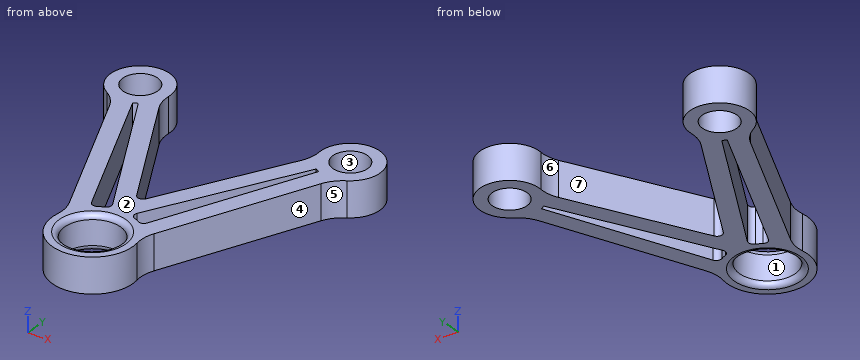
from build123d import *

# Parameters (mm, degrees)
SCHIZZO1_R                   = 5
SCHIZZO1_R_2                 = 8
ESTRUSIONE_ESTRUSIONE1_DEPTH = 5
RACCORDO1_R                  = 10
TAGLIO_ESTRUSIONE1_DEPTH     = 10
RACCORDO2_R                  = 1.5


with BuildPart() as part:
    # Schizzo1 → Estrusione-Estrusione1 (new body, symmetric)
    with BuildSketch(Plane.XY):
        with BuildLine():
            Line((-31.796659285, -8.307948929), (-10.655708964, -56.174972085))
            ThreePointArc((-10.655708964, -56.174972085), (0, -72), (10.655708964, -56.174972085))
            Line((10.655708964, -56.174972085), (31.796659285, -8.307948929))
            ThreePointArc((31.796659285, -8.307948929), (34.104135411, 7.443525544), (22.015418218, -2.914867709))
            Line((22.015418218, -2.914867709), (0, -43.668257767))
            Line((0, -43.668257767), (-22.015418218, -2.914867709))
            ThreePointArc((-22.015418218, -2.914867709), (-34.104135411, 7.443525544), (-31.796659285, -8.307948929))
        make_face()
        with Locations((-30, 0)):
            Circle(SCHIZZO1_R, mode=Mode.SUBTRACT)
        with Locations((30, 0)):
            Circle(SCHIZZO1_R, mode=Mode.SUBTRACT)
        with Locations((0, -60.5)):
            Circle(SCHIZZO1_R_2, mode=Mode.SUBTRACT)
    extrude(amount=ESTRUSIONE_ESTRUSIONE1_DEPTH, both=True)

    # Raccordo1
    raccordo1_edges = [part.edges().sort_by_distance(p)[0] for p in [
        (22.015418218, -2.914867709, 0),
        (31.796659285, -8.307948929, 0),
        (10.655708964, -56.174972085, 0),
        (-10.655708964, -56.174972085, 0),
        (-31.796659285, -8.307948929, 0),
        (-22.015418218, -2.914867709, 0),
    ]]
    fillet(raccordo1_edges, radius=RACCORDO1_R)

    # Schizzo2 → Taglio-Estrusione1 (cut)
    with BuildSketch(Plane.XY.offset(5)):
        with BuildLine():
            Line((-26.565911307, -7.775412198), (-7.229506839, -51.556609655))
            ThreePointArc((-7.229506839, -51.556609655), (-5.059978512, -50.173015084), (-2.637118885, -49.306448107))
            Line((-2.637118885, -49.306448107), (-25.408693659, -7.153314343))
            ThreePointArc((-25.408693659, -7.153314343), (-25.975264878, -7.486755452), (-26.565911307, -7.775412198))
        make_face()
        with BuildLine():
            Line((25.408693659, -7.153314343), (2.637118885, -49.306448107))
            ThreePointArc((2.637118885, -49.306448107), (5.059978512, -50.173015084), (7.229506839, -51.556609655))
            Line((7.229506839, -51.556609655), (26.565911307, -7.775412198))
            ThreePointArc((26.565911307, -7.775412198), (25.975264878, -7.486755452), (25.408693659, -7.153314343))
        make_face()
    extrude(amount=-TAGLIO_ESTRUSIONE1_DEPTH, mode=Mode.SUBTRACT)

    # Raccordo2
    raccordo2_edges = [part.edges().sort_by_distance(p)[0] for p in [
        (-8, -60.5, -5),
        (0, -43.668257767, 0),
        (-8, -60.5, 5),
        (7.229506839, -51.556609655, 0),
        (2.637118885, -49.306448107, 0),
        (-2.637118885, -49.306448107, 0),
        (-7.229506839, -51.556609655, 0),
    ]]
    fillet(raccordo2_edges, radius=RACCORDO2_R)


solid = part.part
Geometry: final body of the model. Coordinates: model frame, mm. Face numbers are marked on the shaded views. A direction names the side the tool comes from. Round coordinates to 2 decimals unless told otherwise and drop trailing zeros. Loops run counter-clockwise (first coordinate to the right, second up) from the corner with the lowest first, then second, coordinate; pieces in that order, holes last. Notation, with made-up numbers: (-37, -25.75) - (21, -25.75) arc R13 ccw to (21, -10.75) - close; hole circle Ø4 at (85.5, 31.5). An arc over 180 degrees is marked (long way). Write each question's results on one line, items separated by ' | '. Start each with the question number.
1) First-contact query: P1, Ø9.5, axis at x = 0, y = -60.5, coming from the -Z side; P2, Ø11.5, axis at x = -30, y = 0, coming from the -Z side; P3, Ø3, axis at y = -17.5, z = 3, coming from the +X side; P4, Ø5, axis at y = -15.5, z = -0.5, coming from the +X side. Flat tips, straight axial feed; report the tip coordinate or a pass-through.
2) Cut plane A-A on x = 0. Return loops of the section in (y, z).
3) Cut plane C-C on y = -40. Return loops of the section in (x, z).
4) Cut plane B-B on y = -60.5. Return loops of the section in (x, z), then the cut area to 3 significant figures.
5) Cut plane D-D on z = -0.25. Count the separate pieces of the cut face and the enclosed holes in it, then the cut area to 3 significant figures.
6) Mould query, pull axis Y, two halves, no side actions, for the marked faces 1, 2, 3 and 4. Classes: released by +Y, released by -Y, zero draft, split by the parting line, or undercut.
7) Access query for the marked faces 5, 6 and 7. Directions: +Z, -Z, +X, -X, +Y, -Y. A direction counts if a zero-diameter tool reaches every point of the face in a straight line with its end or side. Return the directions, or none.
8) Line query: probe 1 along X at (y, z) = (-14, 0); probe 2 along Y at (x, z) = (5, 0.5) (3 decimals); probe 3 along X at (y, z) = (-37, 2). Output: solid intervals per line, ascending. Write a range as [from, to].
Verdict:
1) P1: passes through | P2: stops at z = -5 | P3: stops at x = 28.4 | P4: stops at x = 29.72
2) outline: (-72, -5) - (-70, -5) arc R1.5 ccw to (-68.5, -3.5) - (-68.5, 3.5) arc R1.5 ccw to (-70, 5) - (-72, 5) - close; (-52.5, -3.5) arc R1.5 ccw to (-51, -5) - (-42.01, -5) - (-42.01, 5) - (-51, 5) arc R1.5 ccw to (-52.5, 3.5) - close
3) outline: (-17.8, -5) - (-12.33, -5) - (-12.33, 5) - (-17.8, 5) - close; (-7.66, -5) - (-1.98, -5) - (-1.98, 5) - (-7.66, 5) - close; (1.98, -5) - (7.66, -5) - (7.66, 5) - (1.98, 5) - close; (12.33, -5) - (17.8, -5) - (17.8, 5) - (12.33, 5) - close
4) outline: (-11.5, -5) - (-9.5, -5) arc R1.5 ccw to (-8, -3.5) - (-8, 3.5) arc R1.5 ccw to (-9.5, 5) - (-11.5, 5) - close; (8, -3.5) arc R1.5 ccw to (9.5, -5) - (11.5, -5) - (11.5, 5) - (9.5, 5) arc R1.5 ccw to (8, 3.5) - close | area: 68.1 mm2
5) separate pieces: 1 | enclosed holes: 5 | area: 1,500 mm2
6) face 1: undercut | face 2: zero draft | face 3: undercut | face 4: released by -Y
7) face 5: +Z, -Z, +X, -Y | face 6: +Z, -Z | face 7: +Z, -Z, +Y
8) probe 1: x = [-29.28, -23.82], [-21.71, -16.03], [16.03, 21.71], [23.82, 29.28] | probe 2: y = [-70.856, -66.745], [-54.255, -50.144], [-44.932, -34.413] | probe 3: x = [-19.12, -13.66], [-9.29, -3.6], [3.6, 9.29], [13.66, 19.12]
